Here's the drawing with two shaded views (mm, measured from the low corner). I have some questions. A direction names the side the tool comes from. Round coordinates to 2 decimals unless told otherwise and drop trailing zeros. Order: outer loops, then holes, each group sorted by start corner. A loop starts at its lowest first (then second) coordinate and runs counter-clockwise, first axis right, second up. Notation, with made-up numbers: (53, 21.25) - (84, 21.25) arc R24 cw to (84, 39.25) - close; hole circle Ø4 at (72, 15.25). An arc over 180 degrees is marked (long way). Return JSON: item names as keys, results as strings. Group by question number.
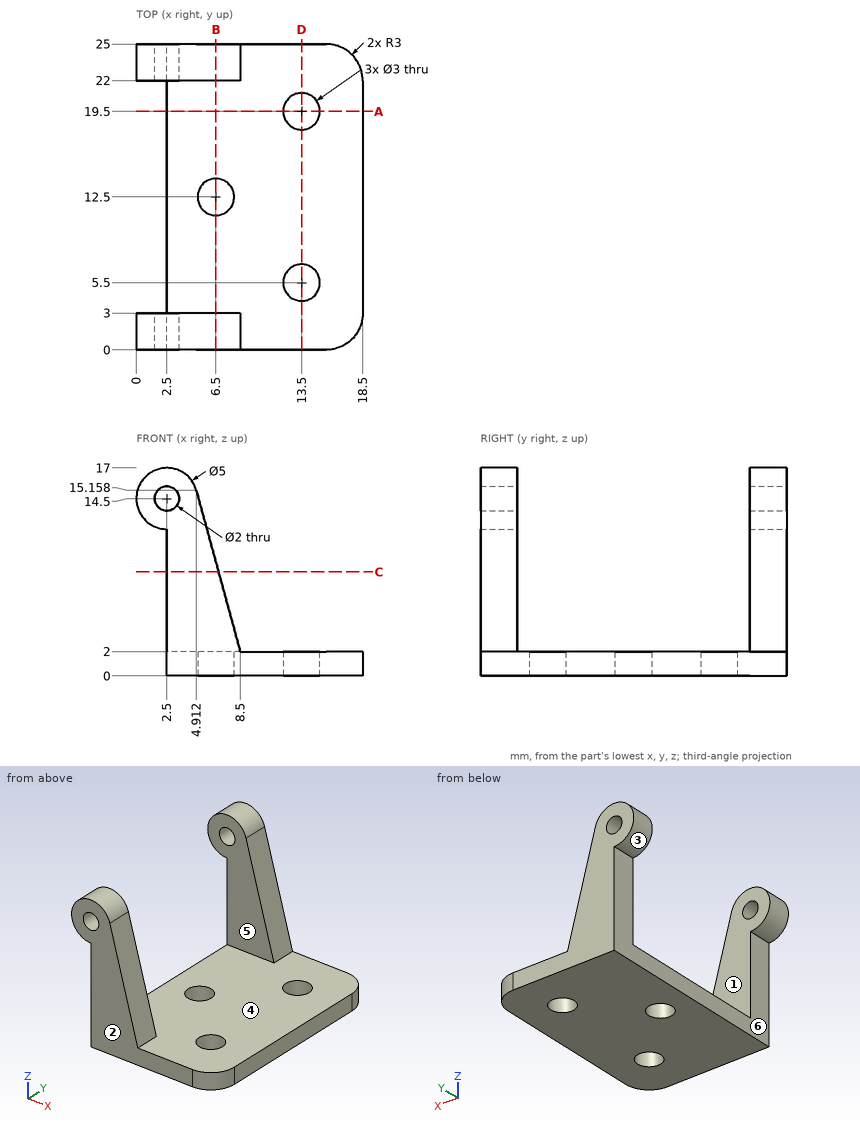
1) For the marked faces 4, 5 and 6, which set-ups out of +Z, -Z, +X, -X, +Y, -Y let a thin tool reach every point of the face, with its end or its side?
2) I want a section at D-D, the plane x = 13.5. List the corners of the cut face in (y, z) for me.
3) If I drill on line 1 along Y through (x, z) = (13.5, 0.5); line 2 along X through (y, z) = (5.5, 1.15); line 3 along X through (y, z) = (12.5, 1.1), over which ranges is the centre line in solid material (lowest first)? Write a range as from..to.
4) We'd pull the mould along Y, two halves only. Please class the marked faces 1, 2 and 3: +Y half, -Y half, draft (parallel to the pull), parting line (faces both ways), or undercut.
5) Will these pins go through, and if not, where does the flat tip stop? pin 1 (3 mm diameter, centred on x = 2.5, z = 14.5, fed in from -Y); pin 2 (1.5 mm diameter, centred on x = 16.5, y = 16.5, fed in from +Z); pin 3 (8 mm diameter, centred on y = 21, z = 14, fed in from +X).
6) I want a section at C-C, the plane z = 8.5. List the corners of the cut face in (x, y) for me.
7) I want a section at B-B, the plane x = 6.5. List the corners of the cut face in (y, z) for me, plus the area to 3 significant figures.
8) I want a section at A-A, the plane y = 19.5. List the corners of the cut face in (x, z) for me.
Outcome:
{
 "1": {"face 4": "+Z, +X", "face 5": "+Z, +X, -X", "face 6": "-Z, -X, +Y, -Y"},
 "2": {"outline": "(0, 0) - (4, 0) - (4, 2) - (0, 2) - close; (7, 0) - (18, 0) - (18, 2) - (7, 2) - close; (21, 0) - (25, 0) - (25, 2) - (21, 2) - close"},
 "3": {"line 1": "0..4, 7..18, 21..25", "line 2": "2.5..12, 15..18.5", "line 3": "2.5..5, 8..18.5"},
 "4": {"face 1": "undercut", "face 2": "-Y half", "face 3": "draft"},
 "5": {"pin 1": "y = 0", "pin 2": "z = 2", "pin 3": "x = 6.28"},
 "6": {"outline": "(2.5, 0) - (6.73, 0) - (6.73, 3) - (2.5, 3) - close; (2.5, 22) - (6.73, 22) - (6.73, 25) - (2.5, 25) - close"},
 "7": {"outline": "(0, 0) - (11, 0) - (11, 2) - (3, 2) - (3, 9.33) - (0, 9.33) - close; (14, 0) - (25, 0) - (25, 9.33) - (22, 9.33) - (22, 2) - (14, 2) - close", "area": "88.0 mm^2"},
 "8": {"outline": "(2.5, 0) - (12, 0) - (12, 2) - (2.5, 2) - close; (15, 0) - (18.5, 0) - (18.5, 2) - (15, 2) - close"}
}
